```python
from build123d import *

# Parameters (mm, degrees)
SKETCH1_R                      = 125
BOSS_EXTRUDE1_DEPTH            = 50
SKETCH2_R                      = 127
SKETCH2_R_2                    = 119
PAKNING_DEPTH                  = 10
SKETCH3_R                      = 125
SKETCH3_R_2                    = 112
PAKNINGSRING_DEPTH             = 3
SKETCH7_R                      = 135
SKETCH7_R_2                    = 115
CUT_EXTRUDE6_DEPTH             = 30
CHAMFER2_SIZE                  = 0.5
CIRPATTERN2_COUNT              = 8
SKETCH19_R                     = 11
SPINDLE_DEPTH                  = 15.5
CIRPATTERN4_COUNT              = 3
F_10_0_10_DIAMETER_HOLE2_D     = 10
F_10_0_10_DIAMETER_HOLE2_DEPTH = 40.5
F_10_0_10_DIAMETER_HOLE2_TIP   = 3.004303095
F_5_0_5_DIAMETER_HOLE2_D       = 5
F_5_0_5_DIAMETER_HOLE2_DEPTH   = 10
F_5_0_5_DIAMETER_HOLE2_TIP     = 1.502151548
F_5_0_5_DIAMETER_HOLE3_D       = 5
F_5_0_5_DIAMETER_HOLE3_DEPTH   = 20.5
F_5_0_5_DIAMETER_HOLE3_TIP     = 1.502151548
M4_TAPPED_HOLE1_AT_2_COUNT     = 2
M4_TAPPED_HOLE1_AT_2_PITCH     = 19
M4_TAPPED_HOLE2_D              = 3.3
M4_TAPPED_HOLE2_DEPTH          = 10.1
M4_TAPPED_HOLE2_TIP            = 0.991420021
M4_TAPPED_HOLE3_D              = 3.3
M4_TAPPED_HOLE3_DEPTH          = 10.1
M4_TAPPED_HOLE3_TIP            = 0.991420021
CIRPATTERN8_COUNT              = 3
CIRPATTERN9_COUNT              = 3
CHAMFER3_SIZE                  = 1


with BuildPart() as part:
    # Sketch1 → Boss-Extrude1 (new body)
    with BuildSketch(Plane(origin=(0, 0, 0), x_dir=(1, 0, 0), z_dir=(0, 1, 0))):
        Circle(SKETCH1_R)
    extrude(amount=BOSS_EXTRUDE1_DEPTH)

    # Sketch2 → Pakning (cut)
    with BuildSketch(Plane(origin=(0, 50, 0), x_dir=(1, 0, 0), z_dir=(0, 1, 0))):
        Circle(SKETCH2_R)
        Circle(SKETCH2_R_2, mode=Mode.SUBTRACT)
    extrude(amount=-PAKNING_DEPTH, mode=Mode.SUBTRACT)

    # Sketch3 → PakningsRing (cut)
    with BuildSketch(Plane(origin=(0, 50, 0), x_dir=(1, 0, 0), z_dir=(0, 1, 0))):
        Circle(SKETCH3_R)
        Circle(SKETCH3_R_2, mode=Mode.SUBTRACT)
    extrude(amount=-PAKNINGSRING_DEPTH, mode=Mode.SUBTRACT)

    # Sketch7 → Cut-Extrude6 (cut)
    with BuildSketch(Plane.XZ):
        Circle(SKETCH7_R)
        Circle(SKETCH7_R_2, mode=Mode.SUBTRACT)
    extrude(amount=-CUT_EXTRUDE6_DEPTH, mode=Mode.SUBTRACT)

    # Chamfer2
    chamfer2_edges = [part.edges().sort_by_distance(p)[0] for p in [
        (-119, 47, 0),
        (-112, 50, 0),
    ]]
    chamfer(chamfer2_edges, length=CHAMFER2_SIZE)

    # Sketch17 → Tapped Hole for M3x0.5 Helicoil1 (revolve, cut)
    with BuildSketch(Plane(origin=(0, 47, -115.5), x_dir=(0, 0, 1), z_dir=(1, 0, 0))):
        Polygon((0, 0), (0, 5.946355475), (1.575, 5), (1.575, 0), align=None)
    tapped_hole_for_m3x0_5_helicoil1 = revolve(axis=Axis((0, 53.35, -115.5), (0, -1, 0)), mode=Mode.SUBTRACT)

    # CirPattern2: Tapped Hole for M3x0.5 Helicoil1 ×8 about axis
    cirpattern2_axis = Axis((0, 0, 0), (0, 1, 0))
    for i in range(1, CIRPATTERN2_COUNT):
        add(tapped_hole_for_m3x0_5_helicoil1.rotate(cirpattern2_axis, i * 360 / CIRPATTERN2_COUNT), mode=Mode.SUBTRACT)

    # Sketch19 → Spindle (cut)
    with BuildSketch(Plane.XZ):
        with Locations((-80, 0)):
            Circle(SKETCH19_R)
    spindle = extrude(amount=-SPINDLE_DEPTH, mode=Mode.SUBTRACT)

    # CirPattern4: Spindle ×3 about axis
    cirpattern4_axis = Axis((0, 0, 0), (0, 1, 0))
    for i in range(1, CIRPATTERN4_COUNT):
        add(spindle.rotate(cirpattern4_axis, i * 360 / CIRPATTERN4_COUNT), mode=Mode.SUBTRACT)

    # Sketch27 → Ø10.0 (10) Diameter Hole1 (revolve, cut)
    with BuildSketch(Plane(origin=(-35, 0, 60.621778265), x_dir=(0, 0, -1), z_dir=(1, 0, 0))):
        Polygon((0, 0), (0, 43.504303095), (5, 40.5), (5, 0), align=None)
    f_10_0_10_diameter_hole1 = revolve(axis=Axis((-35, -6.35, 60.621778265), (0, 1, 0)), mode=Mode.SUBTRACT)

    # Ø10.0 (10) Diameter Hole2
    with Locations(Plane(origin=(0, 0, 0), x_dir=(-1, 0, 0), z_dir=(0, -1, 0))):
        with Locations((0, 0)):
            Hole(F_10_0_10_DIAMETER_HOLE2_D / 2, depth=F_10_0_10_DIAMETER_HOLE2_DEPTH)
            with Locations((0, 0, -(F_10_0_10_DIAMETER_HOLE2_DEPTH + F_10_0_10_DIAMETER_HOLE2_TIP / 2))):  # 118° drill point
                Cone(0, F_10_0_10_DIAMETER_HOLE2_D / 2, F_10_0_10_DIAMETER_HOLE2_TIP, mode=Mode.SUBTRACT)

    # Sketch31 → Ø5.0 (5) Diameter Hole1 (revolve, cut)
    with BuildSketch(Plane(origin=(-35, 50, 60.621778265), x_dir=(0, 0, 1), z_dir=(1, 0, 0))):
        Polygon((0, 0), (0, 11.502151548), (2.5, 10), (2.5, 0), align=None)
    f_5_0_5_diameter_hole1 = revolve(axis=Axis((-35, 56.35, 60.621778265), (0, -1, 0)), mode=Mode.SUBTRACT)

    # Ø5.0 (5) Diameter Hole2
    with Locations(Plane(origin=(0, 50, 0), x_dir=(1, 0, 0), z_dir=(0, 1, 0))):
        with Locations((0, 0)):
            Hole(F_5_0_5_DIAMETER_HOLE2_D / 2, depth=F_5_0_5_DIAMETER_HOLE2_DEPTH)
            with Locations((0, 0, -(F_5_0_5_DIAMETER_HOLE2_DEPTH + F_5_0_5_DIAMETER_HOLE2_TIP / 2))):  # 118° drill point
                Cone(0, F_5_0_5_DIAMETER_HOLE2_D / 2, F_5_0_5_DIAMETER_HOLE2_TIP, mode=Mode.SUBTRACT)

    # Ø5.0 (5) Diameter Hole3
    with Locations(Plane(origin=(0, 0, 0), x_dir=(-1, 0, 0), z_dir=(0, -1, 0))):
        with Locations((-20, -34.641016151)):
            Hole(F_5_0_5_DIAMETER_HOLE3_D / 2, depth=F_5_0_5_DIAMETER_HOLE3_DEPTH)
            with Locations((0, 0, -(F_5_0_5_DIAMETER_HOLE3_DEPTH + F_5_0_5_DIAMETER_HOLE3_TIP / 2))):  # 118° drill point
                Cone(0, F_5_0_5_DIAMETER_HOLE3_D / 2, F_5_0_5_DIAMETER_HOLE3_TIP, mode=Mode.SUBTRACT)

    # Sketch37 → M4 Tapped Hole1 (revolve, cut)
    with BuildSketch(Plane(origin=(-43.227241336, 0, 55.871778265), x_dir=(0, 0, -1), z_dir=(1, 0, 0))):
        Polygon((0, 0), (0, 11.091420021), (1.65, 10.1), (1.65, 0), align=None)
    m4_tapped_hole1 = revolve(axis=Axis((-43.227241336, -6.35, 55.871778265), (0, 1, 0)), mode=Mode.SUBTRACT)

    # M4 Tapped Hole1 at 2: M4 Tapped Hole1 ×2
    with Locations(*[Vector(0.866025404, 0, 0.5) * (i * M4_TAPPED_HOLE1_AT_2_PITCH) for i in range(1, M4_TAPPED_HOLE1_AT_2_COUNT)]):
        add(m4_tapped_hole1, mode=Mode.SUBTRACT)

    # M4 Tapped Hole2
    with Locations(Plane(origin=(0, 0, 0), x_dir=(-1, 0, 0), z_dir=(0, -1, 0))):
        with Locations((8.227241336, -4.75), (-8.227241336, 4.75)):
            Hole(M4_TAPPED_HOLE2_D / 2, depth=M4_TAPPED_HOLE2_DEPTH)
            with Locations((0, 0, -(M4_TAPPED_HOLE2_DEPTH + M4_TAPPED_HOLE2_TIP / 2))):  # 118° drill point
                Cone(0, M4_TAPPED_HOLE2_D / 2, M4_TAPPED_HOLE2_TIP, mode=Mode.SUBTRACT)

    # M4 Tapped Hole3
    with Locations(Plane(origin=(0, 0, 0), x_dir=(-1, 0, 0), z_dir=(0, -1, 0))):
        with Locations((-13.504809472, -38.391016151), (-26.495190528, -30.891016151)):
            Hole(M4_TAPPED_HOLE3_D / 2, depth=M4_TAPPED_HOLE3_DEPTH)
            with Locations((0, 0, -(M4_TAPPED_HOLE3_DEPTH + M4_TAPPED_HOLE3_TIP / 2))):  # 118° drill point
                Cone(0, M4_TAPPED_HOLE3_D / 2, M4_TAPPED_HOLE3_TIP, mode=Mode.SUBTRACT)

    # Sketch43 → Tapped Hole for M5x0.8 Helicoil1 (revolve, cut)
    with BuildSketch(Plane(origin=(52.5, 50, -90.932667397), x_dir=(0, 0, 1), z_dir=(1, 0, 0))):
        Polygon((0, 0), (0, 9.762237609), (2.6, 8.2), (2.6, 0), align=None)
    tapped_hole_for_m5x0_8_helicoil1 = revolve(axis=Axis((52.5, 56.35, -90.932667397), (0, -1, 0)), mode=Mode.SUBTRACT)

    # CirPattern8: Tapped Hole for M5x0.8 Helicoil1 ×3 about axis
    cirpattern8_axis = Axis((0, 0, 0), (0, 1, 0))
    for i in range(1, CIRPATTERN8_COUNT):
        add(tapped_hole_for_m5x0_8_helicoil1.rotate(cirpattern8_axis, i * 360 / CIRPATTERN8_COUNT), mode=Mode.SUBTRACT)

    # CirPattern9: Ø10.0 (10) Diameter Hole1, M4 Tapped Hole1, Ø5.0 (5) Diameter Hole1 ×3 about axis
    cirpattern9_axis = Axis((0, 0, 0), (0, 1, 0))
    for i in range(1, CIRPATTERN9_COUNT):
        add(f_10_0_10_diameter_hole1.rotate(cirpattern9_axis, i * 360 / CIRPATTERN9_COUNT), mode=Mode.SUBTRACT)
        add(m4_tapped_hole1.rotate(cirpattern9_axis, i * 360 / CIRPATTERN9_COUNT), mode=Mode.SUBTRACT)
        add(f_5_0_5_diameter_hole1.rotate(cirpattern9_axis, i * 360 / CIRPATTERN9_COUNT), mode=Mode.SUBTRACT)

    # CirPattern9 copy 1 sketch → CirPattern9 copy 1 (revolve, cut)
    with BuildSketch(Plane(origin=(70, 0, -9.5), x_dir=(-0.866025404, 0, 0.5), z_dir=(-0.5, 0, -0.866025404))):
        Polygon((0, 0), (0, 11.091420021), (1.65, 10.1), (1.65, 0), align=None)
    revolve(axis=Axis((70, -6.35, -9.5), (0, 1, 0)), mode=Mode.SUBTRACT)

    # CirPattern9 copy 2 sketch → CirPattern9 copy 2 (revolve, cut)
    with BuildSketch(Plane(origin=(-43.227241336, 0, -55.871778265), x_dir=(0.866025404, 0, 0.5), z_dir=(-0.5, 0, 0.866025404))):
        Polygon((0, 0), (0, 11.091420021), (1.65, 10.1), (1.65, 0), align=None)
    revolve(axis=Axis((-43.227241336, -6.35, -55.871778265), (0, 1, 0)), mode=Mode.SUBTRACT)

    # Chamfer3
    chamfer3_edges = [part.edges().sort_by_distance(p)[0] for p in [
        (-125, 30, 0),
        (-115, 0, 0),
        (-125, 40, 0),
    ]]
    chamfer(chamfer3_edges, length=CHAMFER3_SIZE)


solid = part.part
```
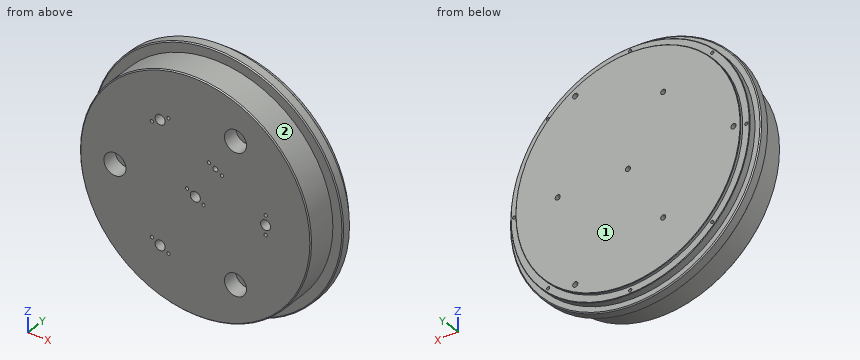
Can you work these out from the model? Positions are in its coordinate system, mm. Face numbers are marked on the shaded views. Give positions to 0.01 mm unless a question says otherwise; leave off trailing zeros. Order: outer loops, then holes, each group sorted by start corner. A loop starts at its lowest first (then second) coordinate and runs counter-clockwise, first axis right, second up. Notation, with made-up numbers: M 10,24 L 29,24 A21 cw 29,57 Z; hole C 83,40 d11. An arc over 180 degrees is marked long. One line per item, written item: value.
1) For P1, Ø4.5, axis at x = 0, z = 0, coming from the +Y side; P2, Ø2, axis at y = 33.5, z = 55.5, coming from the -X side; P3, Ø1.5, axis at y = 44.5, z = -15.5, coming from the +X side; P4, Ø13, axis at x = -80, z = 0, coming from the -Y side, each with a flat end and sliding along its axis, tell me the tip position at first contact or that it passes through.
Answer sheet:
P1: passes through
P2: stops at x = -112.49
P3: stops at x = 118.08
P4: stops at y = 15.5
2) I want a section at A-A, the plane y = 6. Count the separate pieces of the cut face and the enclosed holes in it, plus the area to 3 significant figures.
Answer sheet:
separate pieces: 1
enclosed holes: 18
area: 40,000 mm^2
3) We'd pull the mould along X, two halves only. Please class the marked faces 1 and 2: released by +X, released by -X, zero draft, split by the parting line, or undercut.
Answer sheet:
face 1: zero draft
face 2: split by the parting line
4) I want a section at B-B, the plane y = 35.5. List the corners of the cut face in (x, z) for me.
Answer sheet:
outline: C 0,0 d250; hole C -35,-60.62 d10; hole C -35,60.62 d10; hole C 0,0 d10; hole C 70,0 d10
5) Please list where these lines run through material, in increasing order: line 1 along X through (y, z) = (23, 4); line 2 along Z through (x, y) = (-31.5, 5.5); line 3 along X through (y, z) = (15.5, -15.5).
Answer sheet:
line 1: x = -114.93 to -3, 3 to 67, 73 to 114.93
line 2: z = -110.6 to -64.19, -57.05 to 57.05, 64.19 to 110.6
line 3: x = -113.95 to 113.95
